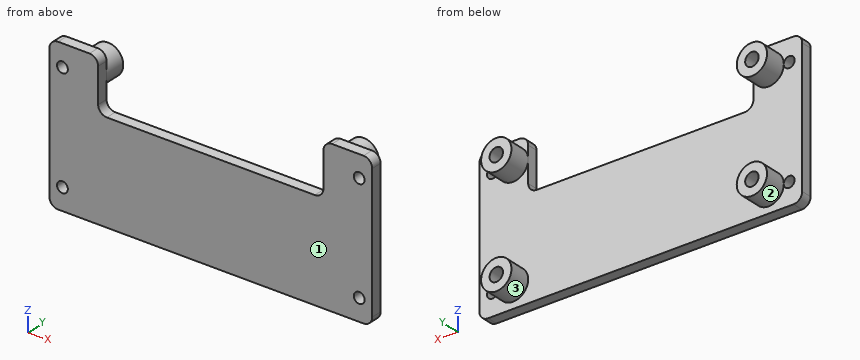
from build123d import *

# Parameters (mm, degrees)
SKETCH1_W           = 94.615
SKETCH1_H           = 44.45
BOSS_EXTRUDE1_DEPTH = 3.175
SKETCH2_R           = 4.445
SKETCH2_R_2         = 1.9685
BOSS_EXTRUDE2_DEPTH = 6.35
SKETCH4_R           = 1.5875
CUT_EXTRUDE1_DEPTH  = 6.35
FILLET1_R           = 2.54
SKETCH6_W           = 66.04
SKETCH6_H           = 15.24
CUT_EXTRUDE2_DEPTH  = 5.08
FILLET2_R           = 2.54


with BuildPart() as part:
    # Sketch1 → Boss-Extrude1 (new body)
    with BuildSketch(Plane(origin=(0, 0, 0), x_dir=(1, 0, 0), z_dir=(0, 1, 0))):
        with Locations((47.3075, 22.225)):
            Rectangle(SKETCH1_W, SKETCH1_H)
    extrude(amount=BOSS_EXTRUDE1_DEPTH)

    # Sketch2 → Boss-Extrude2 (add)
    # profile 1 of 4: a face of its own
    with BuildSketch(Plane(origin=(0, 3.175, 0), x_dir=(1, 0, 0), z_dir=(0, 1, 0))):
        with Locations(Location((9.8425, 6.35, 0), (0, 0, 270))):
            Circle(SKETCH2_R)
        with Locations(Location((9.8425, 6.35, 0), (0, 0, 270))):
            Circle(SKETCH2_R_2, mode=Mode.SUBTRACT)
    # profile 2 of 4: a face of its own
    with BuildSketch(Plane(origin=(0, 3.175, 0), x_dir=(1, 0, 0), z_dir=(0, 1, 0))):
        with Locations(Location((9.8425, 38.1, 0), (0, 0, 270))):
            Circle(SKETCH2_R)
        with Locations(Location((9.8425, 38.1, 0), (0, 0, 270))):
            Circle(SKETCH2_R_2, mode=Mode.SUBTRACT)
    # profile 3 of 4: a face of its own
    with BuildSketch(Plane(origin=(0, 3.175, 0), x_dir=(1, 0, 0), z_dir=(0, 1, 0))):
        with Locations(Location((84.7725, 38.1, 0), (0, 0, 270))):
            Circle(SKETCH2_R)
        with Locations(Location((84.7725, 38.1, 0), (0, 0, 270))):
            Circle(SKETCH2_R_2, mode=Mode.SUBTRACT)
    # profile 4 of 4: a face of its own
    with BuildSketch(Plane(origin=(0, 3.175, 0), x_dir=(1, 0, 0), z_dir=(0, 1, 0))):
        with Locations(Location((84.7725, 6.35, 0), (0, 0, 270))):
            Circle(SKETCH2_R)
        with Locations(Location((84.7725, 6.35, 0), (0, 0, 270))):
            Circle(SKETCH2_R_2, mode=Mode.SUBTRACT)
    extrude(amount=BOSS_EXTRUDE2_DEPTH)

    # Sketch4 → Cut-Extrude1 (cut)
    with BuildSketch(Plane(origin=(0, 3.175, 0), x_dir=(1, 0, 0), z_dir=(0, 1, 0))):
        with Locations(Location((3.81, 38.1, 0), (0, 0, 270))):
            Circle(SKETCH4_R)
        with Locations(Location((3.81, 6.35, 0), (0, 0, 270))):
            Circle(SKETCH4_R)
        with Locations(Location((90.805, 38.1, 0), (0, 0, 270))):
            Circle(SKETCH4_R)
        with Locations(Location((90.805, 6.35, 0), (0, 0, 270))):
            Circle(SKETCH4_R)
    extrude(amount=-CUT_EXTRUDE1_DEPTH, mode=Mode.SUBTRACT)

    # Fillet1
    fillet1_edges = [part.edges().sort_by_distance(p)[0] for p in [
        (0, 1.5875, -44.45),
        (0, 1.5875, 0),
        (94.615, 1.5875, 0),
        (94.615, 1.5875, -44.45),
    ]]
    fillet(fillet1_edges, radius=FILLET1_R)

    # Sketch6 → Cut-Extrude2 (cut)
    with BuildSketch(Plane(origin=(0, 3.175, 0), x_dir=(1, 0, 0), z_dir=(0, 1, 0))):
        with Locations((47.3075, 7.62)):
            Rectangle(SKETCH6_W, SKETCH6_H)
    extrude(amount=-CUT_EXTRUDE2_DEPTH, mode=Mode.SUBTRACT)

    # Fillet2
    fillet2_edges = [part.edges().sort_by_distance(p)[0] for p in [
        (14.2875, 1.5875, 0),
        (14.2875, 1.5875, -15.24),
        (80.3275, 1.5875, -15.24),
        (80.3275, 1.5875, 0),
    ]]
    fillet(fillet2_edges, radius=FILLET2_R)


solid = part.part
Work out the finished part from the listing and answer in its coordinate system (mm). Face numbers are marked on the shaded views. Give positions to 0.01 mm unless a question says otherwise; leave off trailing zeros. Loops run counter-clockwise (first coordinate to the right, second up) from the corner with the lowest first, then second, coordinate; pieces in that order, holes last. Notation, with made-up numbers: (-38.5, 41.5) - (-25.5, 41.5) arc R10 ccw to (-25.5, 49.5) - close; hole circle Ø5 at (31.5, 67.25). An arc over 180 degrees is marked (long way). Answer in a Markdown table with one row per item. Add a question column.
Q1. The part is cut by section D-D (x = 47). Determine the outline of the cut face in (y, z) (3 decimals), and give its area (3 significant figures).
Q2. The part is cut by section A-A (x = 3.81). State how many separate pieces and enclosed holes the cut face has, and give its area (3 significant figures).
Q3. Determine the mould class of the marked faces 1, 2 and 3 for opening direction X: released by +X, released by -X, zero draft, split by the parting line, or undercut.
Q4. Each of these flat-tipped pins is pushed along its axis until it touches: P1, Ø3, axis at x = 85, z = -38, coming from the +Y side (3 decimals); P2, Ø1.6, axis at x = 40, y = 2, coming from the +Z side. Where does it stop, or does it pass through?
Q5. Consider line 1 along Z through (x, y) = (3.81, 1.8); line 2 along X through (y, z) = (2.15, -38.1) (1 decimal); line 3 along X through (y, z) = (8.25, -38.1). Determine where each line is inside the solid, lowest interval first.
Q6. The part is cut by section C-C (z = -24.5). Determine the outline of the cut face in (x, y) (3 decimals), and give its area (3 significant figures).
Solution:
| question | item | result |
|---|---|---|
| 1 | outline | (0, -44.45) - (3.175, -44.45) - (3.175, -15.24) - (0, -15.24) - close |
| 1 | area | 92.7 mm² |
| 2 | separate pieces | 3 |
| 2 | enclosed holes | 0 |
| 2 | area | 121 mm² |
| 3 | face 1 | zero draft |
| 3 | face 2 | undercut |
| 3 | face 3 | undercut |
| 4 | P1 | stops at y = 3.175 |
| 4 | P2 | stops at z = -15.24 |
| 5 | line 1 | z = -44.45 to -39.69, -36.51 to -7.94, -4.76 to 0 |
| 5 | line 2 | x = 0 to 2.2, 5.4 to 89.2, 92.4 to 94.6 |
| 5 | line 3 | x = 5.4 to 7.87, 11.81 to 14.29, 80.33 to 82.8, 86.74 to 89.22 |
| 6 | outline | (0, 0) - (94.615, 0) - (94.615, 3.175) - (0, 3.175) - close |
| 6 | area | 300 mm² |
